```python
from build123d import *

# Parameters (mm, degrees)
F0_R            = 23.01875
F0_R_2          = 2.15265
F0_R_3          = 11.1125
F1_DEPTH        = 3.175
F3_DEPTH        = 3.175
F3_COPIES_COUNT = 4


# Not quite as in the source:
# - a pattern or mirror of a feature is missing from the dataset's text; its kind, count and spacing are read off the source's solid


with BuildPart() as f1:
    # F0 (on Top) → F1 (new body)
    with BuildSketch(Plane.XY):
        Circle(F0_R)
        with Locations((-12.3478521665, -12.3478521665)):
            Circle(F0_R_2, mode=Mode.SUBTRACT)
        with Locations((12.3478521665, -12.3478521665)):
            Circle(F0_R_2, mode=Mode.SUBTRACT)
        with Locations((-12.3478521665, 12.3478521665)):
            Circle(F0_R_2, mode=Mode.SUBTRACT)
        Circle(F0_R_3, mode=Mode.SUBTRACT)
        with Locations((12.3478521665, 12.3478521665)):
            Circle(F0_R_2, mode=Mode.SUBTRACT)
    extrude(amount=F1_DEPTH)

    # F2 (on face) → F3 (cut, through all)
    with BuildSketch(Plane.XY.offset(3.175)):
        with BuildLine():
            ThreePointArc((-9.7719120136, 17.2709047146), (-7.6525973796, 15.318794197), (-6.7959542154, 12.5677230456))
            ThreePointArc((-6.7959542154, 12.5677230456), (0, 14.2875), (6.7959542154, 12.5677230456))
            ThreePointArc((6.7959542154, 12.5677230456), (7.6525973796, 15.318794197), (9.7719120136, 17.2709047146))
            ThreePointArc((9.7719120136, 17.2709047146), (0, 19.84375), (-9.7719120136, 17.2709047146))
        make_face()
    f3 = extrude(amount=-F3_DEPTH, mode=Mode.SUBTRACT)

    # F3_copies: F3 ×4 about axis
    f3_copies_axis = Axis((0, 0, 0), (0, 0, 1))
    for i in range(1, F3_COPIES_COUNT):
        add(f3.rotate(f3_copies_axis, i * 360 / F3_COPIES_COUNT), mode=Mode.SUBTRACT)


solid = f1.part
```
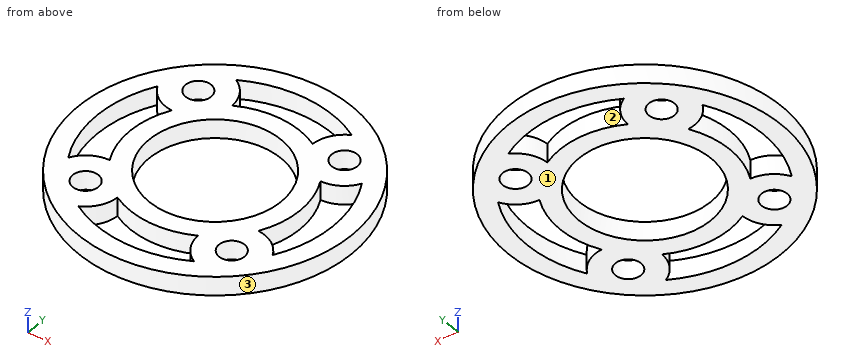
Source: CAD feature listing. Evaluate the final solid. Frame: model axes, mm. Face numbers are marked on the shaded views. Coordinates: 2 decimals unless noted, no trailing zeros. Loops run counter-clockwise (first coordinate to the right, second up) from the corner with the lowest first, then second, coordinate; pieces in that order, holes last. Notation, with made-up numbers: M -11,87 L 8,87 A18 ccw 8,105 Z; hole C -7,40.5 d5. An arc over 180 degrees is marked long. Use CSV: the item, a comma, the result in double quotes.
(1) Line query: line 1 (X direction, y = -1.5, z = 0.75); line 2 (X direction, y = 1, z = 1.1); line 3 (Y direction, x = 9, z = 1). Output: solid intervals per line, ascending. Write a range as [from, to].
Answers follow:
line 1,"[-22.97, -19.79], [-14.21, -11.01], [11.01, 14.21], [19.79, 22.97]"
line 2,"[-23, -19.82], [-14.25, -11.07], [11.07, 14.25], [19.82, 23]"
line 3,"[-21.19, -17.69], [-16.78, -6.52], [6.52, 16.78], [17.69, 21.19]"
(2) Cut plane D-D on x = 12. Return loops of the section in (y, z) (1 decimal).
Answers follow:
outline,"M -19.6,0 L -14.5,0 L -14.5,3.2 L -19.6,3.2 Z; M -10.2,0 L 10.2,0 L 10.2,3.2 L -10.2,3.2 Z; M 14.5,0 L 19.6,0 L 19.6,3.2 L 14.5,3.2 Z"
(3) Cut plane B-B on x = 2.5. Return loops of the section in (y, z) (3 decimals).
Answers follow:
outline,"M -22.883,0 L -19.686,0 L -19.686,3.175 L -22.883,3.175 Z; M -14.067,0 L -10.828,0 L -10.828,3.175 L -14.067,3.175 Z; M 10.828,0 L 14.067,0 L 14.067,3.175 L 10.828,3.175 Z; M 19.686,0 L 22.883,0 L 22.883,3.175 L 19.686,3.175 Z"
(4) Draft query along X for the marked faces 1, 2 and 3. Return one class per face: pulls with the +X half, pulls with the -X half, needs draft (parallel to the pull), parting line crosses it, or undercut.
Answers follow:
face 1,"needs draft"
face 2,"undercut"
face 3,"parting line crosses it"
(5) Cut plane A-A on y = 0. Return loops of the section in (x, z) (1 decimal).
Answers follow:
outline,"M -23,0 L -19.8,0 L -19.8,3.2 L -23,3.2 Z; M -14.3,0 L -11.1,0 L -11.1,3.2 L -14.3,3.2 Z; M 11.1,0 L 14.3,0 L 14.3,3.2 L 11.1,3.2 Z; M 19.8,0 L 23,0 L 23,3.2 L 19.8,3.2 Z"
(6) Contact query for flat-ended pins moving along their axis: pin 1 (1.5 mm diameter, centred on x = -7.5, z = 2.5, fed in from -Y); pin 2 (4 mm diameter, centred on x = 12.35, y = 12.35, fed in from +Z); pin 3 (1.5 mm diameter, centred on y = 3, z = 3, fed in from +X). Output: stop coordinate, or through.
Answers follow:
pin 1,"y = -22.01"
pin 2,"through"
pin 3,"x = 22.91"
(7) Cut plane C-C on z = 1.9. Give the number of separate pieces and of enclosed holes in the cut face, and give its area (3 significant figures).
Answers follow:
separate pieces,"1"
enclosed holes,"9"
area,"856 mm²"
